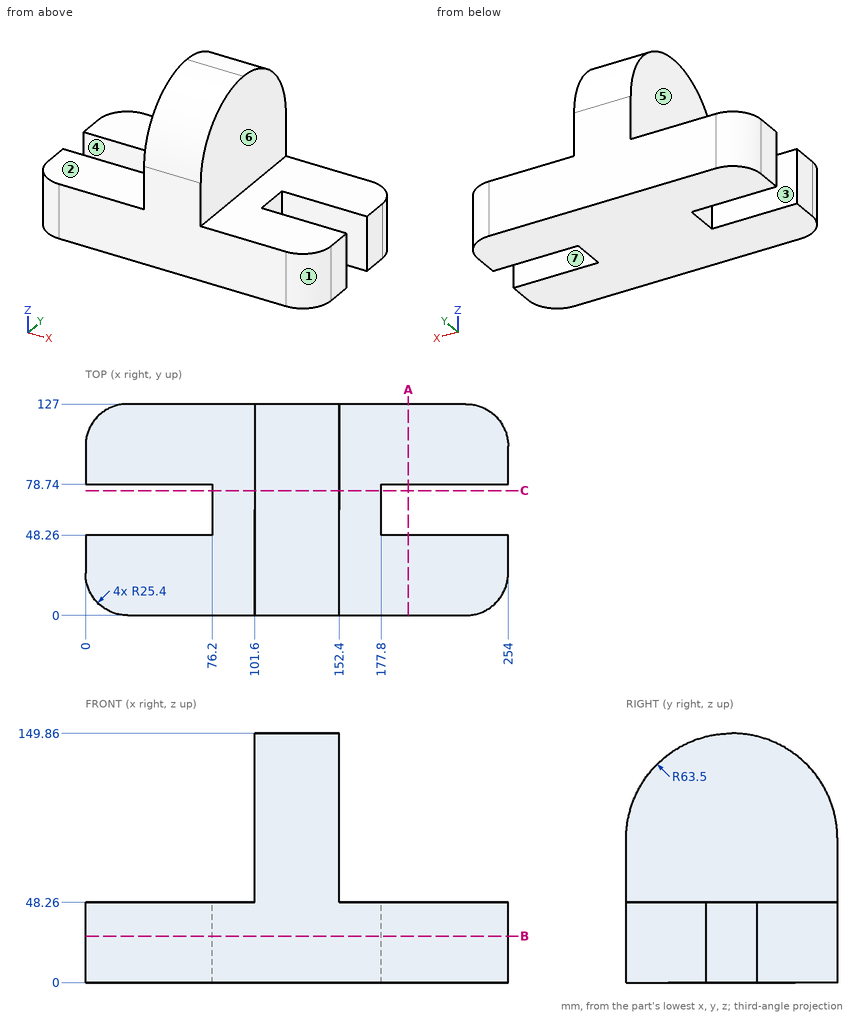
Study the drawing (mm; zero at the part's minimum x, y, z) and answer. A direction names the side the tool comes from. Give positions to 0.01 mm unless a question says otherwise; leave off trailing zeros. Write each loop counter-clockwise with the first axis right and the second up, starting at its lowest first coordinate (ties: lowest second). Pieces come first, ordered by that corner, then holes. Notation, with made-up numbers: (74.25, 30.5) - (79.25, 30.5) arc R22 cw to (79.25, 53.5) - close; hole circle Ø4 at (28.5, 29). An arc over 180 degrees is marked (long way). Use a Markdown table: item, result.
1. For a pull along Y with two mould halves and no side action, classify the marked faces 1, 2 and 3 as released by +Y, released by -Y, zero draft, split by the parting line, or undercut.
Values follow:
| item | result |
|---|---|
| face 1 | released by -Y |
| face 2 | zero draft |
| face 3 | undercut |
2. Find the intervals of material crossed by probe 1 along X at (y, z) = (68, 80); probe 2 along Z at (x, y) = (161.5, 89.5); probe 3 along Y at (x, z) = (227, 32.5), in increasing order. Write a range as from..to.
Values follow:
| item | result |
|---|---|
| probe 1 | x = 101.6..152.4 |
| probe 2 | z = 0..48.26 |
| probe 3 | y = 0..48.26, 78.74..127 |
3. Section C-C on y = 75 is taken. Write down the section's boundary in (x, z).
Values follow:
| item | result |
|---|---|
| outline | (76.2, 0) - (177.8, 0) - (177.8, 48.26) - (152.4, 48.26) - (152.4, 148.81) - (101.6, 148.81) - (101.6, 48.26) - (76.2, 48.26) - close |
4. Section A-A on x = 194 is taken. Write down the section's boundary in (y, z), plus the area to 3 significant figures.
Values follow:
| item | result |
|---|---|
| outline | (0, 0) - (48.26, 0) - (48.26, 48.26) - (0, 48.26) - close; (78.74, 0) - (127, 0) - (127, 48.26) - (78.74, 48.26) - close |
| area | 4,660 mm² |
5. Section B-B on z = 28 is taken. Write down the section's boundary in (x, y), plus the area to 3 significant figures.
Values follow:
| item | result |
|---|---|
| outline | (0, 25.4) arc R25.4 ccw to (25.4, 0) - (228.6, 0) arc R25.4 ccw to (254, 25.4) - (254, 48.26) - (177.8, 48.26) - (177.8, 78.74) - (254, 78.74) - (254, 101.6) arc R25.4 ccw to (228.6, 127) - (25.4, 127) arc R25.4 ccw to (0, 101.6) - (0, 78.74) - (76.2, 78.74) - (76.2, 48.26) - (0, 48.26) - close |
| area | 27,100 mm² |
6. A tool of negligible diameter and unlimited length cuts with its end or side. For the marked faces 4, 5, 6 and 7, from which of +Z, -Z, +X, -X, +Y, -Y can it reach the whole face along a straight path? Write none if from no direction.
Values follow:
| item | result |
|---|---|
| face 4 | +Z, -Z, -X |
| face 5 | +Z, -X, +Y, -Y |
| face 6 | +Z, +X, +Y, -Y |
| face 7 | +Z, -Z, +X |
7. Each of these flat-tipped pins is pushed along its axis until it touches: P1, Ø15, axis at y = 58.5, z = 24.5, coming from the -X side; P2, Ø4, axis at y = 23.5, z = 122.5, coming from the +X side; P3, Ø4, axis at x = 153.5, y = 66.5, coming from the +Z side; P4, Ø1, axis at x = 100.5, z = 121, coming from the -Y side. Where does it stop, or does it pass through?
Values follow:
| item | result |
|---|---|
| P1 | stops at x = 76.2 |
| P2 | stops at x = 152.4 |
| P3 | stops at z = 149.85 |
| P4 | passes through |
